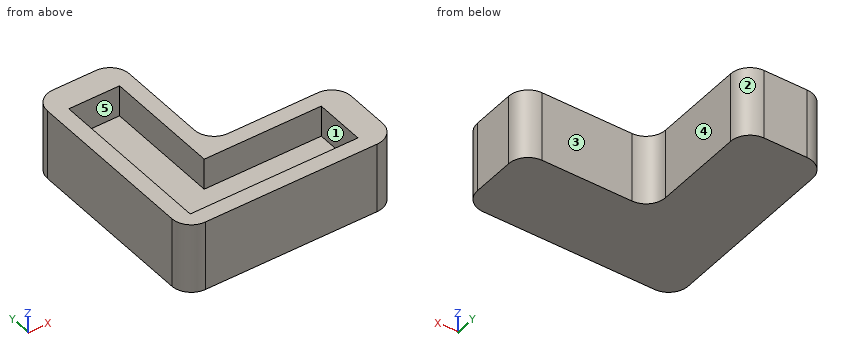
```python
from build123d import *

# Parameters (mm, degrees)
F1_DEPTH = 18
F2_DEPTH = 10
F3_R     = 5


with BuildPart() as f1:
    # F0 (on Top) → F1 (new body)
    with BuildSketch(Plane.XY):
        Polygon((0, 54), (0, 0), (54, 0), (54, 4), (47, 4), (4, 4), (4, 47), (4, 54), align=None)
        Polygon((47, 4), (54, 4), (54, 21), (21, 21), (21, 54), (4, 54), (4, 47), (17, 47), (17, 17), (47, 17), align=None)
    extrude(amount=F1_DEPTH)

    # F0 (on Top) → F2 (join)
    with BuildSketch(Plane.XY):
        Polygon((4, 4), (47, 4), (47, 17), (17, 17), (17, 47), (4, 47), align=None)
    extrude(amount=F2_DEPTH)

    # F3
    f3_edges = [f1.edges().sort_by_distance(p)[0] for p in [
        (0, 0, 9),
        (0, 54, 9),
        (54, 0, 9),
        (54, 21, 9),
        (21, 54, 9),
        (21, 21, 9),
    ]]
    fillet(f3_edges, radius=F3_R)


solid = f1.part
```
The listing builds one solid part. Answer for the finished solid, in the listing's coordinates (mm). Face numbers are marked on the shaded views. A direction names the side the tool comes from. Round coordinates to 2 decimals unless told otherwise and drop trailing zeros. Loops run counter-clockwise (first coordinate to the right, second up) from the corner with the lowest first, then second, coordinate; pieces in that order, holes last. Notation, with made-up numbers: (20.25, 8) - (56.25, 8) arc R18 cw to (56.25, 14) - close; hole circle Ø8 at (-11, 21). An arc over 180 degrees is marked (long way). Return JSON: item names as keys, results as strings. Group by question number.
1. The part is cut by section B-B on x = 15. Determine the outline of the cut face in (y, z), then the cut area to 3 significant figures.
2. The mould has two halves that part along X. Classify the marked faces 3, 4 and 5: pulls with the +X half, pulls with the -X half, needs draft (parallel to the pull), parting line crosses it, or undercut.
3. The part is cut by section D-D on z = 15.25. Determine the outline of the cut face in (x, y).
4. Consider probe 1 along X at (y, z) = (26, 15); probe 2 along Y at (x, z) = (16, 11). Determine where each line is inside the solid, lowest interval first.
5. Each of these flat-tipped pins is pushed along its axis until it touches: P1, Ø5.5, axis at y = 37, z = 8, coming from the +X side; P2, Ø2, axis at x = 36, z = 11.5, coming from the +Y side; P3, Ø2.5, axis at x = 21, z = 14.5, coming from the +Y side; P4, Ø8, axis at x = 28.5, y = 48.5, coming from the +Z side. Where does it stop, or does it pass through?
6. Which of the six approach directions +Z, -Z, +X, -X, +Y, -Y give full straight-line access (tool end or side, diameter ignored) to the marked faces 1 and 2?
7. The part is cut by section A-A on z = 2.5. Determine the outline of the cut face in (x, y), then the cut area to 3 significant figures.
Resolved:
{
 "1": {"outline": "(0, 0) - (54, 0) - (54, 18) - (47, 18) - (47, 10) - (4, 10) - (4, 18) - (0, 18) - close", "area": "628 mm²"},
 "2": {"face 3": "needs draft", "face 4": "pulls with the +X half", "face 5": "undercut"},
 "3": {"outline": "(0, 5) arc R5 ccw to (5, 0) - (49, 0) arc R5 ccw to (54, 5) - (54, 16) arc R5 ccw to (49, 21) - (26, 21) arc R5 cw to (21, 26) - (21, 49) arc R5 ccw to (16, 54) - (5, 54) arc R5 ccw to (0, 49) - close; hole (4, 4) - (47, 4) - (47, 17) - (17, 17) - (17, 47) - (4, 47) - close"},
 "4": {"probe 1": "x = 0 to 4, 17 to 21", "probe 2": "y = 0 to 4, 47 to 54"},
 "5": {"P1": "stops at x = 21", "P2": "stops at y = 21", "P3": "stops at y = 52.31", "P4": "passes through"},
 "6": {"face 1": "+Z", "face 2": "+Z, -Z, +X, +Y"},
 "7": {"outline": "(0, 5) arc R5 ccw to (5, 0) - (49, 0) arc R5 ccw to (54, 5) - (54, 16) arc R5 ccw to (49, 21) - (26, 21) arc R5 cw to (21, 26) - (21, 49) arc R5 ccw to (16, 54) - (5, 54) arc R5 ccw to (0, 49) - close", "area": "1,810 mm²"}
}
